Read the model definition and answer for the solid it produces. Units are mm, in the model's axes. Face numbers are marked on the shaded views. A direction names the side the tool comes from. Coordinates: 2 decimals unless noted, no trailing zeros. Loops run counter-clockwise (first coordinate to the right, second up) from the corner with the lowest first, then second, coordinate; pieces in that order, holes last. Notation, with made-up numbers: (4, 14) -> (18, 14) arc R11 cw to (18, 27) -> close; hole circle Ø4 at (78.25, 10). An arc over 180 degrees is marked (long way). One line per question, with ' | ' between items. Start each with the question number.
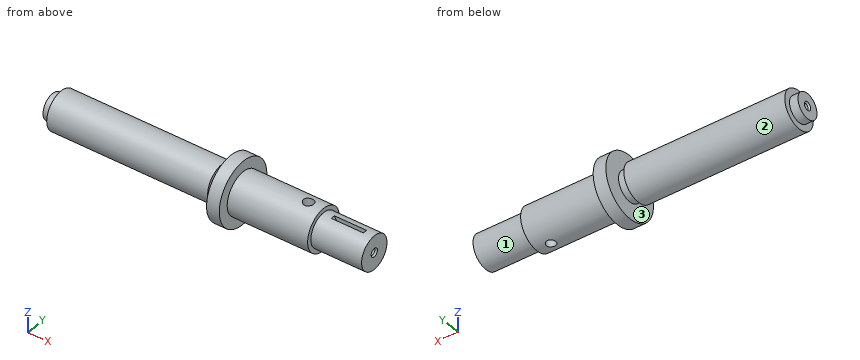
```python
from build123d import *

# Parameters (mm, degrees)
F1_R                 = 6.35
F6_DEPTH             = 0.79375
F4_D                 = 2.38125
F4_DEPTH             = 3.175
F4_CSINK_D           = 3.14325
F4_CSINK_ANGLE       = 60
F4_TIP               = 0.7153996745
F4_ON_F8_D           = 2.38125
F4_ON_F8_DEPTH       = 3.175
F4_ON_F8_CSINK_D     = 3.14325
F4_ON_F8_CSINK_ANGLE = 60
F4_ON_F8_TIP         = 0.7153996745


with BuildPart() as f0:
    # F5 (on Front) → F0 (revolve)
    with BuildSketch(Plane.XZ):
        Polygon((-60.325, -3.175), (-60.325, -7.9375), (60.325, -7.9375), (60.325, -1.5875), (41.275, -1.5875), (41.275, 0), (11.1125, 0), (11.1125, 3.96875), (6.35, 3.96875), (6.35, -2.38125), (3.175, -2.38125), (3.175, -0.79375), (-57.15, -0.79375), (-57.15, -3.175), align=None)
    revolve(axis=Axis((0, 0, -7.9375), (1, 0, 0)))

    # F1 (on Front) → F6 (cut, symmetric)
    with BuildSketch(Plane.XZ):
        with Locations((50.8, 0.396875)):
            Circle(F1_R)
    extrude(amount=F6_DEPTH, both=True, mode=Mode.SUBTRACT)

    # F2 (on Front) → F7 (revolve, cut)
    with BuildSketch(Plane.XZ):
        with BuildLine():
            Line((37.43325, -20.3236020014), (37.69995, 4.3383559637))
            ThreePointArc((37.69995, 4.3383559637), (36.7317963469, 4.6552760961), (35.71875, 4.7625))
            Line((35.71875, 4.7625), (35.71875, -20.6375))
            ThreePointArc((35.71875, -20.6375), (36.5902490252, -20.5583786828), (37.43325, -20.3236020014))
        make_face()
    revolve(axis=Axis((35.71875, 0, 0), (0, 0, -1)), mode=Mode.SUBTRACT)

    # F4
    with Locations(Plane.YZ.offset(60.325)):
        with Locations((0, -7.9375)):
            CounterSinkHole(F4_D / 2, F4_CSINK_D / 2, depth=F4_DEPTH, counter_sink_angle=F4_CSINK_ANGLE)
            with Locations((0, 0, -(F4_DEPTH + F4_TIP / 2))):  # 118° drill point
                Cone(0, F4_D / 2, F4_TIP, mode=Mode.SUBTRACT)

    # F4 on F8
    with Locations(Plane(origin=(-60.325, 0, 0), x_dir=(0, -1, 0), z_dir=(-1, 0, 0))):
        with Locations((0, -7.9375)):
            CounterSinkHole(F4_ON_F8_D / 2, F4_ON_F8_CSINK_D / 2, depth=F4_ON_F8_DEPTH, counter_sink_angle=F4_ON_F8_CSINK_ANGLE)
            with Locations((0, 0, -(F4_ON_F8_DEPTH + F4_ON_F8_TIP / 2))):  # 118° drill point
                Cone(0, F4_ON_F8_D / 2, F4_ON_F8_TIP, mode=Mode.SUBTRACT)


solid = f0.part
```
(1) Each of these flat-tipped pins is pushed along its axis until it touches: pin 1 Ø12 at (x, z) = (42.5, -8.5) entering from -Y; pin 2 Ø5 at (x, y) = (-36, -5.5) entering from -Z; pin 3 Ø1.5 at (y, z) = (0, -16.5) entering from +X (3 decimals); pin 4 Ø5 at (y, z) = (-0.5, -8.5) entering from -X (3 decimals). Where does it stop, or does it pass through?
(2) Section C-C on y = 9 is taken. Write down the section's boundary in (x, z).
(3) Find the intervals of material crossed by probe 1 along X at (y, z) = (-5.75, -7.5) (3 decimals); probe 2 along Z at (x, y) = (-58.95, 0) (3 decimals); probe 3 along X at (y, z) = (-5.5, -11.25) (3 decimals), in increasing order. Write a range as from..to.
(4) Section D-D on x = 14 is taken. Write down the section's boundary in (y, z) (1 decimal).
(5) A tool of negligible diameter and unlimited length cuts with its end or side. For the marked faces 1, 2 and 3, from which of +Z, -Z, +X, -X, +Y, -Y can it reach the whole face along a straight path? Write none if from no direction.
(6) Section B-B on x = -38 is taken. Write down the section's boundary in (y, z), plus the area to 3 significant figures.
Working result:
1) pin 1: stops at y = -7.94 | pin 2: stops at z = -14.42 | pin 3: stops at x = 41.275 | pin 4: stops at x = -60.325
2) outline: (6.35, -15.73) -> (11.11, -15.73) -> (11.11, -0.14) -> (6.35, -0.14) -> close
3) probe 1: x = -57.15..3.175, 6.35..60.325 | probe 2: z = -12.7..-9.128, -6.747..-3.175 | probe 3: x = -57.15..3.175, 6.35..41.275
4) outline: circle Ø15.9 at (0, -7.9)
5) face 1: +X | face 2: -X | face 3: none
6) outline: circle Ø14.29 at (0, -7.94) | area: 160 mm2
